```python
from build123d import *

# Parameters (mm, degrees)
SKETCH1_W           = 12.5
SKETCH1_H           = 5.9
BOSS_EXTRUDE1_DEPTH = 7
SKETCH3_W           = 11
SKETCH3_H           = 4
CUT_EXTRUDE1_DEPTH  = 5
SKETCH4_W           = 1.2
SKETCH4_H           = 3.5
CUT_EXTRUDE2_DEPTH  = 4
SKETCH5_W           = 12.5
SKETCH5_H           = 0.8
CUT_EXTRUDE3_DEPTH  = 0.8
SKETCH6_W           = 0.8
SKETCH6_H           = 0.8
CUT_EXTRUDE4_DEPTH  = 10
SKETCH7_W           = 11
SKETCH7_H           = 1
CUT_EXTRUDE5_DEPTH  = 0.3


with BuildPart() as part:
    # Sketch1 → Boss-Extrude1 (new body)
    with BuildSketch(Plane(origin=(0, 0, 0), x_dir=(1, 0, 0), z_dir=(0, 1, 0))):
        Rectangle(SKETCH1_W, SKETCH1_H)
    extrude(amount=BOSS_EXTRUDE1_DEPTH)

    # Sketch3 → Cut-Extrude1 (cut)
    with BuildSketch(Plane.XZ):
        Rectangle(SKETCH3_W, SKETCH3_H)
    extrude(amount=-CUT_EXTRUDE1_DEPTH, mode=Mode.SUBTRACT)

    # Sketch4 → Cut-Extrude2 (cut)
    with BuildSketch(Plane.XY.offset(2.95)):
        with Locations((-3.58, 1.75)):
            Rectangle(SKETCH4_W, SKETCH4_H)
        with Locations((3.22, 1.75)):
            Rectangle(SKETCH4_W, SKETCH4_H)
    extrude(amount=-CUT_EXTRUDE2_DEPTH, mode=Mode.SUBTRACT)

    # Sketch5 → Cut-Extrude3 (cut)
    with BuildSketch(Plane(origin=(0, 7, 0), x_dir=(1, 0, 0), z_dir=(0, 1, 0))):
        with Locations((0, 2.55)):
            Rectangle(SKETCH5_W, SKETCH5_H)
    extrude(amount=-CUT_EXTRUDE3_DEPTH, mode=Mode.SUBTRACT)

    # Sketch6 → Cut-Extrude4 (cut)
    with BuildSketch(Plane(origin=(0, 7, 0), x_dir=(1, 0, 0), z_dir=(0, 1, 0))):
        with Locations((3.8, -0.55)):
            Rectangle(SKETCH6_W, SKETCH6_H)
        with Locations((1.266666667, -0.55)):
            Rectangle(SKETCH6_W, SKETCH6_H)
        with Locations((-1.266666667, -0.55)):
            Rectangle(SKETCH6_W, SKETCH6_H)
        with Locations((-3.8, -0.55)):
            Rectangle(SKETCH6_W, SKETCH6_H)
    extrude(amount=-CUT_EXTRUDE4_DEPTH, mode=Mode.SUBTRACT)

    # Sketch7 → Cut-Extrude5 (cut)
    with BuildSketch(Plane.XZ.offset(-5)):
        with Locations((0, -1.5)):
            Rectangle(SKETCH7_W, SKETCH7_H)
    extrude(amount=-CUT_EXTRUDE5_DEPTH, mode=Mode.SUBTRACT)


solid = part.part
```
For this review, take the finished solid that the model builds, in its own axes (mm). A direction names the side the tool comes from. Round coordinates to 2 decimals unless told otherwise and drop trailing zeros. Write each loop counter-clockwise with the first axis right and the second up, starting at its lowest first coordinate (ties: lowest second). Pieces come first, ordered by that corner, then holes. Notation, with made-up numbers: (32.25, 64.5) - (41.25, 64.5) arc R18 cw to (41.25, 71.5) - close; hole circle Ø1 at (-18.75, 72.5). An arc over 180 degrees is marked (long way). Put each result on its own line as item: value.
Q1. We need section A-A (x = -1.5). Give the boundary of the cut face in (y, z).
Solved:
outline: (0, -2.95) - (6.2, -2.95) - (6.2, -2.15) - (7, -2.15) - (7, 0.15) - (5, 0.15) - (5, -1) - (5.3, -1) - (5.3, -2) - (0, -2) - close; (0, 2) - (5, 2) - (5, 0.95) - (7, 0.95) - (7, 2.95) - (0, 2.95) - close
Q2. We need section D-D (y = 3). Give the boundary of the cut face in (x, z), and give its area (3 significant figures).
Solved:
outline: (-6.25, -2.95) - (6.25, -2.95) - (6.25, 2.95) - (3.82, 2.95) - (3.82, 2) - (5.5, 2) - (5.5, -2) - (-5.5, -2) - (-5.5, 2) - (-4.18, 2) - (-4.18, 2.95) - (-6.25, 2.95) - close; (-2.98, 2) - (2.62, 2) - (2.62, 2.95) - (-2.98, 2.95) - close
area: 27.5 mm2
Q3. Machinability: for faces 4 (the face through (4, 6, 0.15)), 5 (the face through (-5.5, 3, 0)), 6 (the face through (-3.6, 3.5, 2.5)), which of the approach directions +Z, -Z, +X, -X, +Y, -Y give a long, thin tool a straight path to every point of the face, cutting with its end or side? Answer none if there is none.
Solved:
face 4: +Y, -Y
face 5: -Y
face 6: +Z, -Y
Q4. We need section B-B (z = 0.6). Give the boundary of the cut face in (x, y), and give its area (3 significant figures).
Solved:
outline: (-6.25, 0) - (-5.5, 0) - (-5.5, 5) - (-4.2, 5) - (-4.2, 7) - (-6.25, 7) - close; (-3.4, 5) - (-1.67, 5) - (-1.67, 7) - (-3.4, 7) - close; (-0.87, 5) - (0.87, 5) - (0.87, 7) - (-0.87, 7) - close; (1.67, 5) - (3.4, 5) - (3.4, 7) - (1.67, 7) - close; (4.2, 5) - (5.5, 5) - (5.5, 0) - (6.25, 0) - (6.25, 7) - (4.2, 7) - close
area: 26.1 mm2
Q5. Mouldability with a two-part tool opening along X and no side actions: class faces 1 (the face through (6.25, 3, 0)), 2 (the face through (0, 5, 1)), 3 (the face through (0, 3, 2.95)) as released by +X, released by -X, zero draft, split by the parting line, or undercut.
Solved:
face 1: released by +X
face 2: undercut
face 3: zero draft
Q6. We need section C-C (y = 4.5). Give the boundary of the cut face in (x, z), and give its area (4 significant figures).
Solved:
outline: (-6.25, -2.95) - (6.25, -2.95) - (6.25, 2.95) - (-6.25, 2.95) - close; hole (-5.5, -2) - (5.5, -2) - (5.5, 2) - (-5.5, 2) - close
area: 29.75 mm2
Q7. Insertion check: pin 1 Ø1.5 at (x, z) = (1, 1) entering from -Y; pin 2 Ø3 at (x, z) = (-1.5, -2) entering from -Y. Each pin has a flat end and moves straight along its axis. Give the tip position at first contact, or say it passes through.
Solved:
pin 1: stops at y = 5
pin 2: stops at y = 0
Q8. Wall thickness on probe 1 along Z at (x, y) = (-3.75, 6.5); probe 2 along Z at (x, y) = (-1, 0.75); probe 3 along X at (y, z) = (3.25, 0.45): over which ranges is each line inside the solid? List them lowest first.
Solved:
probe 1: z = -2.15 to 0.15, 0.95 to 2.95
probe 2: z = -2.95 to -2, 2 to 2.95
probe 3: x = -6.25 to -5.5, 5.5 to 6.25
